Read the model definition and answer for the solid it produces. Units are mm, in the model's axes. A direction names the side the tool comes from. Coordinates: 2 decimals unless noted, no trailing zeros. Loops run counter-clockwise (first coordinate to the right, second up) from the corner with the lowest first, then second, coordinate; pieces in that order, holes last. Notation, with made-up numbers: (22, 3) - (80, 3) arc R14 ccw to (80, 25) - close; hole circle Ø3 at (-39, 30). An arc over 180 degrees is marked (long way). One line per question, with ' | ' between items. Start each with the question number.
```python
from build123d import *

# Parameters (mm, degrees)
SKETCH2_W           = 80
SKETCH2_H           = 40
BOSS_EXTRUDE1_DEPTH = 7.5
SKETCH3_W           = 80
SKETCH3_H           = 18.5
CUT_EXTRUDE1_DEPTH  = 5
SKETCH9_W           = 80
SKETCH9_H           = 16.5
CUT_EXTRUDE5_DEPTH  = 5
SKETCH10_W          = 20
SKETCH10_H          = 40
CUT_EXTRUDE7_DEPTH  = 10
SKETCH12_W          = 40
SKETCH12_H          = 20
CUT_EXTRUDE8_DEPTH  = 10
SKETCH13_W          = 60
SKETCH13_H          = 5
BOSS_EXTRUDE5_DEPTH = 10
SKETCH14_W          = 60
SKETCH14_H          = 5
BOSS_EXTRUDE6_DEPTH = 5
SKETCH15_R          = 2.5
BOSS_EXTRUDE7_DEPTH = 30


with BuildPart() as part:
    # Sketch2 → Boss-Extrude1 (new body)
    with BuildSketch(Plane(origin=(0, 0, 0), x_dir=(0, 0, -1), z_dir=(1, 0, 0))):
        with Locations((0, 20)):
            Rectangle(SKETCH2_W, SKETCH2_H)
    extrude(amount=BOSS_EXTRUDE1_DEPTH)

    # Sketch3 → Cut-Extrude1 (cut)
    with BuildSketch(Plane(origin=(7.5, 0, 0), x_dir=(0, 0, -1), z_dir=(1, 0, 0))):
        with Locations((0, 9.25)):
            Rectangle(SKETCH3_W, SKETCH3_H)
    extrude(amount=-CUT_EXTRUDE1_DEPTH, mode=Mode.SUBTRACT)

    # Sketch9 → Cut-Extrude5 (cut)
    with BuildSketch(Plane(origin=(7.5, 0, 0), x_dir=(0, 0, -1), z_dir=(1, 0, 0))):
        with Locations((0, 26.75)):
            Rectangle(SKETCH9_W, SKETCH9_H)
    extrude(amount=-CUT_EXTRUDE5_DEPTH, mode=Mode.SUBTRACT)

    # Sketch10 → Cut-Extrude7 (cut)
    with BuildSketch(Plane.ZY):
        with Locations((-30, 20)):
            Rectangle(SKETCH10_W, SKETCH10_H)
    extrude(amount=-CUT_EXTRUDE7_DEPTH, mode=Mode.SUBTRACT)

    # Sketch12 → Cut-Extrude8 (cut)
    with BuildSketch(Plane.ZY):
        with Locations((10, 20)):
            Rectangle(SKETCH12_W, SKETCH12_H)
    extrude(amount=-CUT_EXTRUDE8_DEPTH, mode=Mode.SUBTRACT)

    # Sketch13 → Boss-Extrude5 (add)
    with BuildSketch(Plane(origin=(2.5, 0, 0), x_dir=(0, 0, -1), z_dir=(1, 0, 0))):
        with Locations((-10, 32.5)):
            Rectangle(SKETCH13_W, SKETCH13_H)
    extrude(amount=BOSS_EXTRUDE5_DEPTH)

    # Sketch14 → Boss-Extrude6 (add)
    with BuildSketch(Plane(origin=(7.5, 0, 0), x_dir=(0, 0, -1), z_dir=(1, 0, 0))):
        with Locations((-10, 37.5)):
            Rectangle(SKETCH14_W, SKETCH14_H)
    extrude(amount=BOSS_EXTRUDE6_DEPTH)

    # Sketch15 → Boss-Extrude7 (add)
    with BuildSketch(Plane(origin=(2.5, 0, 0), x_dir=(0, 0, -1), z_dir=(1, 0, 0))):
        with Locations((-22.5, 5)):
            Circle(SKETCH15_R)
        with Locations((2.5, 5)):
            Circle(SKETCH15_R)
    extrude(amount=BOSS_EXTRUDE7_DEPTH)


solid = part.part
```
1) Which of the six approach directions +Z, -Z, +X, -X, +Y, -Y give full straight-line access (tool end or side, diameter ignored) to faces 1 (the cylindrical face through (17, 5, 25)), 2 (the flat face through (2, 29, -20)), 3 (the flat face through (12.5, 35, 10)), 4 (the flat face through (1, 20, 30))?
2) The part is cut by section C-C on x = 10. Write down the section's boundary in (y, z).
3) The part is cut by section A-A on y = 19. Write down the section's boundary in (x, z), and give its area (3 significant figures).
4) The mould has two halves that part along Z. Classify faces 5 (the flat face through (6, 30, 10)), 6 (the cylindrical face through (17, 7, -1)), 7 (the flat face through (0, 34, 10)), 8 (the flat face through (2, 29, 40)): released by +Z, released by -Z, zero draft, split by the parting line, or undercut.
5) The part is cut by section D-D on y = 5. Write down the section's boundary in (x, z), and give its area (3 significant figures).
6) Find the intervals of material crossed by line 1 along Y through (x, z) = (6.5, 2.5); line 2 along X through (y, z) = (7, 2); line 3 along X through (y, z) = (35.5, 20), in increasing order. Write a range as from..to.
7) Given pin 1 Ø8 at (x, z) = (28, -6) entering from +Y; pin 2 Ø11 at (y, z) = (35.5, 7.5) entering from +X; pin 3 Ø6 at (x, z) = (23.5, 15) entering from +Y; pin 4 Ø10 at (x, y) = (26.5, 10) entering from +Z, each flat-ended and moving along its own axis, determine where each tip first touches the part or whether it passes through.
8) The part is cut by section B-B on z = 12. Write down the section's boundary in (x, y).
Answer below:
1) face 1: +X | face 2: -Z, +X, -X, +Y, -Y | face 3: +Z, -Z, +X, +Y | face 4: +X, -X
2) outline: circle Ø5 at (5, -2.5); circle Ø5 at (5, 22.5); (30, -20) - (40, -20) - (40, 40) - (30, 40) - close
3) outline: (0, -20) - (2.5, -20) - (2.5, -10) - (0, -10) - close; (0, 30) - (2.5, 30) - (2.5, 40) - (0, 40) - close | area: 50.0 mm2
4) face 5: undercut | face 6: undercut | face 7: zero draft | face 8: released by +Z
5) outline: (0, -20) - (2.5, -20) - (2.5, -5) - (32.5, -5) - (32.5, 0) - (2.5, 0) - (2.5, 20) - (32.5, 20) - (32.5, 25) - (2.5, 25) - (2.5, 40) - (0, 40) - close | area: 450 mm2
6) line 1: 30..40 | line 2: 0..2.5 | line 3: 0..12.5
7) pin 1: y = 7.5 | pin 2: x = 12.5 | pin 3: through | pin 4: z = 25
8) outline: (0, 0) - (2.5, 0) - (2.5, 10) - (0, 10) - close; (0, 30) - (12.5, 30) - (12.5, 40) - (0, 40) - close
